Input: dimensioned drawing with shaded views. Units: mm. Origin: part minimum x, y, z. Coordinates: 2 decimals unless noted, no trailing zeros. Order: outer loops, then holes, each group sorted by start corner. A loop starts at its lowest first (then second) coordinate and runs counter-clockwise, first axis right, second up.
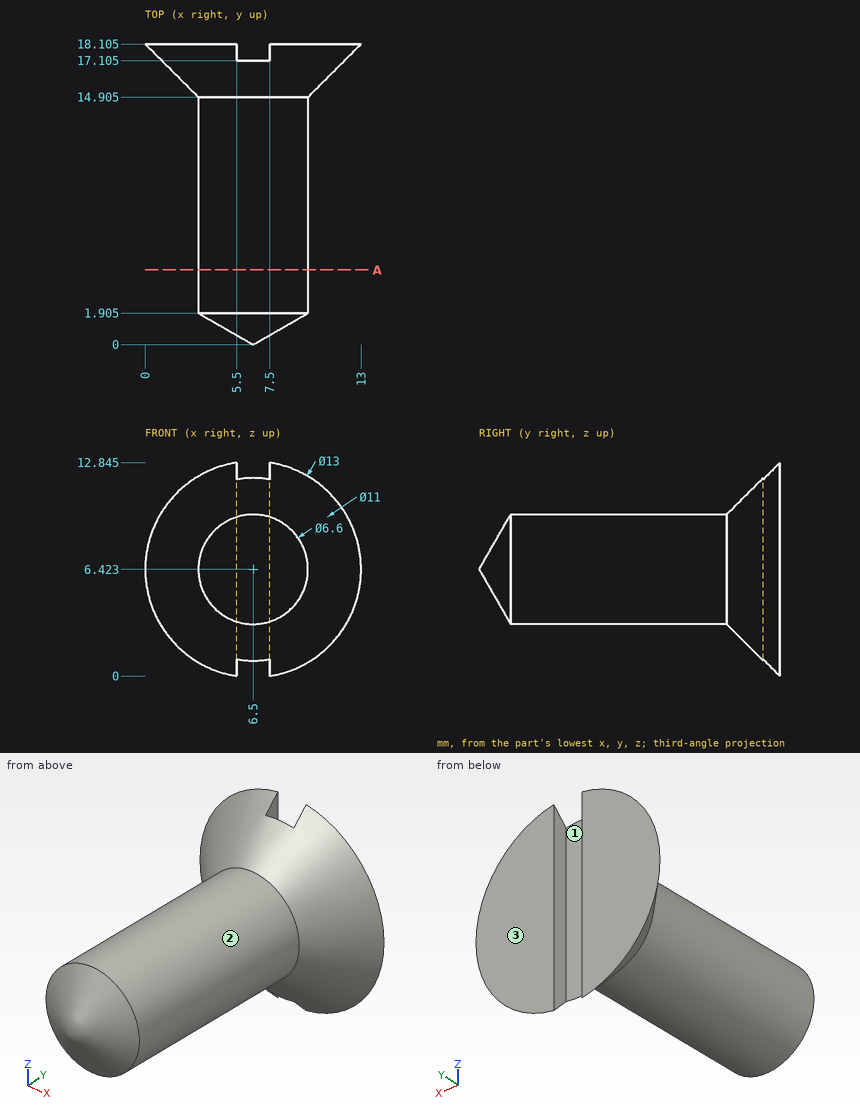
1. Pin query (flat end, axial travel): P1, Ø2, axis at y = 16, z = 1.5, coming from the +X side (1 decimal); P2, Ø3, axis at x = 1.5, y = 2.5, coming from the -Z side; P3, Ø3, axis at x = 2, y = 12.5, coming from the +Z side (1 decimal); P4, Ø5, axis at x = 3, z = 3, coming from the -Y side. Return the tip coordinate at first contact, or that it passes through.
Findings:
P1: stops at x = 9.4
P2: passes through
P3: stops at z = 7.8
P4: stops at y = 1.38
2. Draft query along X for the marked faces 1, 2 and 3. Return one class per face: released by +X, released by -X, zero draft, split by the parting line, or undercut.
Findings:
face 1: undercut
face 2: split by the parting line
face 3: zero draft
3. Section query A-A on y = 4.5. Return loops of the section in (x, z), plus the area to 3 significant figures.
Findings:
outline: circle Ø6.6 at (6.5, 6.42)
area: 34.2 mm2
4. Ray query, line 1 (X direction, y = 9.5, z = 5); line 2 (X direction, y = 14.5, z = 4.25) (1 decimal); line 3 (Y direction, x = 4.5, z = 2.25) (1 decimal). Return the intervals inside material, ascending.
Findings:
line 1: x = 3.52 to 9.48
line 2: x = 4 to 9
line 3: y = 16.2 to 18.1
